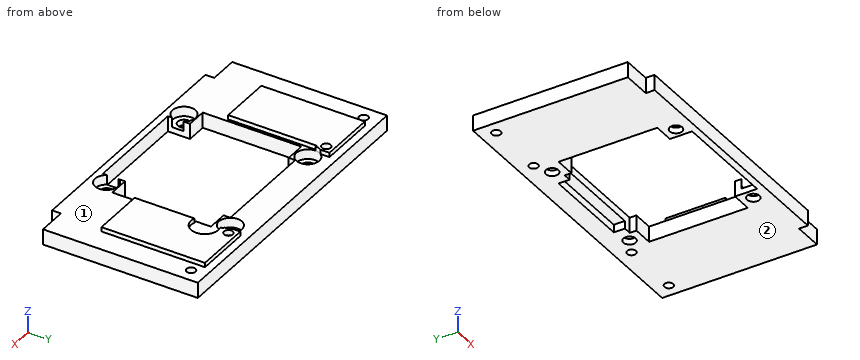
```python
from build123d import *

# Parameters (mm, degrees)
SKETCH3_R           = 1.4
SKETCH3_R_2         = 1
BOSS_EXTRUDE1_DEPTH = 3.5
SKETCH9_R           = 2.6
CUT_EXTRUDE1_DEPTH  = 2.2
SKETCH10_W          = 20
SKETCH10_H          = 2.5
CUT_EXTRUDE2_DEPTH  = 1.75
SKETCH11_R          = 1
BOSS_EXTRUDE2_DEPTH = 1
SKETCH14_R          = 3.1
CUT_EXTRUDE3_DEPTH  = 1
SKETCH15_W          = 6.5
SKETCH15_H          = 2
CUT_EXTRUDE4_DEPTH  = 53.08126138


with BuildPart() as part:
    # Sketch3 → Boss-Extrude1 (new body)
    with BuildSketch(Plane.XY):
        Polygon((-37.436821352, -0.962627815), (-37.436821352, 36.037372185), (31.003178648, 36.037372185), (31.003178648, -0.962627815), (7.298178648, -0.962627815), (-14.831821352, -0.962627815), align=None)
        with Locations((-17.216821352, 30.777902568)):
            Circle(SKETCH3_R, mode=Mode.SUBTRACT)
        with Locations((-34.436821352, 32.642902568)):
            Circle(SKETCH3_R_2, mode=Mode.SUBTRACT)
        with Locations((-20.926821352, 32.642902568)):
            Circle(SKETCH3_R_2, mode=Mode.SUBTRACT)
        with Locations((14.493178648, 32.642902568)):
            Circle(SKETCH3_R_2, mode=Mode.SUBTRACT)
        with Locations((28.003178648, 32.642902568)):
            Circle(SKETCH3_R_2, mode=Mode.SUBTRACT)
        with Locations((-17.216821352, 2.777902568)):
            Circle(SKETCH3_R, mode=Mode.SUBTRACT)
        with Locations((10.783178648, 30.777902568)):
            Circle(SKETCH3_R, mode=Mode.SUBTRACT)
        with Locations((10.783178648, 2.777902568)):
            Circle(SKETCH3_R, mode=Mode.SUBTRACT)
        Polygon((-14.981821352, 0.537372185), (-14.981821352, 5.537372185), (-19.581821352, 5.537372185), (-19.581821352, 27.842902568), (-14.981821352, 27.842902568), (-14.981821352, 29.342902568), (8.548178648, 29.342902568), (8.548178648, 27.842902568), (13.148178648, 27.842902568), (13.148178648, 5.537372185), (8.548178648, 5.537372185), (8.548178648, 0.537372185), align=None, mode=Mode.SUBTRACT)
    extrude(amount=BOSS_EXTRUDE1_DEPTH)

    # Sketch9 → Cut-Extrude1 (cut)
    with BuildSketch(Plane(origin=(0, 0, 3.5), x_dir=(-1, 0, 0), z_dir=(0, 0, -1))):
        with Locations((-10.783178648, 30.777902568)):
            Circle(SKETCH9_R)
        with Locations((17.216821352, 30.777902568)):
            Circle(SKETCH9_R)
        with Locations((-10.783178648, 2.777902568)):
            Circle(SKETCH9_R)
        with Locations((17.216821352, 2.777902568)):
            Circle(SKETCH9_R)
    extrude(amount=CUT_EXTRUDE1_DEPTH, mode=Mode.SUBTRACT)

    # Sketch10 → Cut-Extrude2 (cut)
    with BuildSketch(Plane(origin=(0, 0, 0), x_dir=(-1, 0, 0), z_dir=(0, 0, -1))):
        with Locations((3.216821352, 30.592902568)):
            Rectangle(SKETCH10_W, SKETCH10_H)
    extrude(amount=-CUT_EXTRUDE2_DEPTH, mode=Mode.SUBTRACT)

    # Sketch11 → Boss-Extrude2 (add)
    with BuildSketch(Plane.XY.offset(3.5)):
        with BuildLine():
            Line((-32.136821352, 30.942902568), (-32.136821352, 10.942902568))
            Line((-32.136821352, 10.942902568), (-20.136821352, 10.942902568))
            Line((-20.136821352, 10.942902568), (-20.136821352, 30.942902568))
            Line((-20.136821352, 30.942902568), (-19.811580493, 30.942902568))
            ThreePointArc((-19.811580493, 30.942902568), (-19.664705899, 31.654179489), (-19.326821352, 32.297079977))
            Line((-19.326821352, 32.297079977), (-19.326821352, 34.342902568))
            Line((-19.326821352, 34.342902568), (-32.136821352, 34.342902568))
            Line((-32.136821352, 34.342902568), (-32.136821352, 30.942902568))
        make_face()
        with Locations((-20.926821352, 32.642902568)):
            Circle(SKETCH11_R, mode=Mode.SUBTRACT)
    boss_extrude2 = extrude(amount=BOSS_EXTRUDE2_DEPTH)

    # Mirror1: Boss-Extrude2 across plane
    add(boss_extrude2.mirror(Plane.ZY.offset(3.216821352)))

    # Sketch14 → Cut-Extrude3 (cut)
    with BuildSketch(Plane.XY.offset(4.5)):
        with Locations((14.642214959, 27.392343087)):
            Circle(SKETCH14_R)
    extrude(amount=-CUT_EXTRUDE3_DEPTH, mode=Mode.SUBTRACT)

    # Sketch15 → Cut-Extrude4 (cut, through all)
    with BuildSketch(Plane.XY.offset(3.5)):
        with Locations((-34.186821352, 0.037372185)):
            Rectangle(SKETCH15_W, SKETCH15_H)
        with Locations((27.753178648, 0.037372185)):
            Rectangle(SKETCH15_W, SKETCH15_H)
    extrude(amount=-CUT_EXTRUDE4_DEPTH, mode=Mode.SUBTRACT)


solid = part.part
```
Source: CAD feature listing. Evaluate the final solid. Frame: model axes, mm. Face numbers are marked on the shaded views. Round coordinates to 2 decimals unless told otherwise and drop trailing zeros. Loops run counter-clockwise (first coordinate to the right, second up) from the corner with the lowest first, then second, coordinate; pieces in that order, holes last. Notation, with made-up numbers: M -9.5,31.5 L 0.5,31.5 A12 cw 0.5,38.5 Z; hole C 11.25,-7.5 d4. An arc over 180 degrees is marked long. Use a Markdown table: item, result. Add a question column.
1. Section query D-D on z = 2.6. Give the number of separate pieces and of enclosed holes in the cut face, then the cut area to 3 significant figures.
2. Section query A-A on y = 13.5. Return the cut outline in (x, z).
3. Section query C-C on x = -25. Return the cut outline in (y, z).
4. Mould query, pull axis X, two halves, no side actions, for the marked faces 1 and 2. Classes: pulls with the +X half, pulls with the -X half, needs draft (parallel to the pull), parting line crosses it, or undercut.
5. Contact query for flat-ended pins moving along their axis: P1, Ø4, axis at x = -17.22, y = 30.78, coming from the +Z side; P2, Ø0.5, axis at y = 30.5, z = 4, coming from the -X side; P3, Ø6, axis at x = -7, y = 27, coming from the +Z side. Output: stop coordinate, or through.
6. Line query: line 1 (Y direction, x = -14, z = 0.7); line 2 (X direction, y = 11, z = 2.8); line 3 (X direction, y = 29, z = 1). Output: solid intervals per line, ascending.
7. Section query B-B on x = -4. Return the cut outline in (y, z).
Reported:
| question | item | result |
|---|---|---|
| 1 | separate pieces | 1 |
| 1 | enclosed holes | 7 |
| 1 | area | 1,530 mm² |
| 2 | outline | M -37.44,0 L -19.58,0 L -19.58,3.5 L -20.14,3.5 L -20.14,4.5 L -32.14,4.5 L -32.14,3.5 L -37.44,3.5 Z; M 13.15,0 L 31,0 L 31,3.5 L 25.7,3.5 L 25.7,4.5 L 13.7,4.5 L 13.7,3.5 L 13.15,3.5 Z |
| 3 | outline | M -0.96,0 L 36.04,0 L 36.04,3.5 L 34.34,3.5 L 34.34,4.5 L 10.94,4.5 L 10.94,3.5 L -0.96,3.5 Z |
| 4 | face 1 | undercut |
| 4 | face 2 | needs draft |
| 5 | P1 | stops at z = 1.3 |
| 5 | P2 | stops at x = -32.14 |
| 5 | P3 | stops at z = 3.5 |
| 6 | line 1 | y = -0.96 to 0.54, 29.34 to 36.04 |
| 6 | line 2 | x = -37.44 to -19.58, 13.15 to 31 |
| 6 | line 3 | x = -37.44 to -14.98, 8.55 to 31 |
| 7 | outline | M -0.96,0 L 0.54,0 L 0.54,3.5 L -0.96,3.5 Z; M 29.34,1.75 L 31.84,1.75 L 31.84,0 L 36.04,0 L 36.04,3.5 L 29.34,3.5 Z |
